```python
from build123d import *

# Parameters (mm, degrees)
CROQUIS1_R              = 2.4
CROQUIS1_R_2            = 2.1
SALIENTE_EXTRUIR1_DEPTH = 0.2
CROQUIS3_R              = 5.6
CROQUIS3_R_2            = 2.3
SALIENTE_EXTRUIR2_DEPTH = 0.1
CROQUIS5_R              = 2.4
CROQUIS5_R_2            = 2.1
SALIENTE_EXTRUIR3_DEPTH = 5


with BuildPart() as part:
    # Croquis1 → Saliente-Extruir1 (new body)
    with BuildSketch(Plane(origin=(0, 0, 0), x_dir=(1, 0, 0), z_dir=(0, 1, 0))):
        Circle(CROQUIS1_R)
        Circle(CROQUIS1_R_2, mode=Mode.SUBTRACT)
    saliente_extruir1 = extrude(amount=SALIENTE_EXTRUIR1_DEPTH)



with BuildPart() as body_2:
    # Croquis3 → Saliente-Extruir2 (new body)
    with BuildSketch(Plane.XZ):
        Circle(CROQUIS3_R)
        Circle(CROQUIS3_R_2, mode=Mode.SUBTRACT)
    saliente_extruir2 = extrude(amount=SALIENTE_EXTRUIR2_DEPTH)


with BuildPart() as part_1:
    add(part.part)

    add(body_2.part)  # Saliente-Extruir3 merges body 2
    # Croquis5 → Saliente-Extruir3 (add)
    with BuildSketch(Plane.XZ):
        Circle(CROQUIS5_R)
        Circle(CROQUIS5_R_2, mode=Mode.SUBTRACT)
    saliente_extruir3 = extrude(amount=SALIENTE_EXTRUIR3_DEPTH)

    # Simetría2: Saliente-Extruir1, Saliente-Extruir2, Saliente-Extruir3 across plane
    add(saliente_extruir1.mirror(Plane(origin=(0, -5, 0), x_dir=(0, 0, 1), z_dir=(0, -1, 0))))
    add(saliente_extruir2.mirror(Plane(origin=(0, -5, 0), x_dir=(0, 0, 1), z_dir=(0, -1, 0))))
    add(saliente_extruir3.mirror(Plane(origin=(0, -5, 0), x_dir=(0, 0, 1), z_dir=(0, -1, 0))))


solid = part_1.part
```
Input: part model. Units: mm. Frame: model coordinates. Coordinates: 2 decimals unless noted, no trailing zeros. Loops run counter-clockwise (first coordinate to the right, second up) from the corner with the lowest first, then second, coordinate; pieces in that order, holes last.
Q1. Contact query for flat-ended pins moving along their axis: pin 1 (3 mm diameter, centred on y = -8, z = -0.5, fed in from -X); pin 2 (4 mm diameter, centred on x = -3, y = -2.5, fed in from +Z); pin 3 (2 mm diameter, centred on x = -0.5, y = -6, fed in from -Z). Output: stop coordinate, or through.
Results are:
pin 1: stops at x = -2.4
pin 2: stops at z = 2.18
pin 3: stops at z = -2.4
Q2. Section A-A, the plane z = 0. Return the cut outline in (x, y), and give its area (3 significant figures).
Results are:
outline: (-5.6, -10) - (-2.4, -10) - (-2.4, -10.2) - (-2.1, -10.2) - (-2.1, 0.2) - (-2.4, 0.2) - (-2.4, 0) - (-5.6, 0) - (-5.6, -0.1) - (-2.4, -0.1) - (-2.4, -9.9) - (-5.6, -9.9) - close; (2.1, -10.2) - (2.4, -10.2) - (2.4, -10) - (5.6, -10) - (5.6, -9.9) - (2.4, -9.9) - (2.4, -0.1) - (5.6, -0.1) - (5.6, 0) - (2.4, 0) - (2.4, 0.2) - (2.1, 0.2) - close
area: 7.52 mm2
Q3. Section D-D, the plane z = 1.5. Return the cut outline in (x, y), and give its area (3 significant figures).
Results are:
outline: (-5.4, -10) - (-1.87, -10) - (-1.87, -10.2) - (-1.47, -10.2) - (-1.47, 0.2) - (-1.87, 0.2) - (-1.87, 0) - (-5.4, 0) - (-5.4, -0.1) - (-1.87, -0.1) - (-1.87, -9.9) - (-5.4, -9.9) - close; (1.47, -10.2) - (1.87, -10.2) - (1.87, -10) - (5.4, -10) - (5.4, -9.9) - (1.87, -9.9) - (1.87, -0.1) - (5.4, -0.1) - (5.4, 0) - (1.87, 0) - (1.87, 0.2) - (1.47, 0.2) - close
area: 9.81 mm2
Q4. Section B-B, the plane x = -4.5. Return the cut outline in (y, z), and give its area (3 significant figures).
Results are:
outline: (-10, -3.33) - (-9.9, -3.33) - (-9.9, 3.33) - (-10, 3.33) - close; (-0.1, -3.33) - (0, -3.33) - (0, 3.33) - (-0.1, 3.33) - close
area: 1.33 mm2
Q5. Line query: line 1 along X through (y, z) = (-7.25, 0); line 2 along Z through (x, y) = (-0.5, -6). Output: solid intervals per line, ascending.
Results are:
line 1: x = -2.4 to -2.1, 2.1 to 2.4
line 2: z = -2.35 to -2.04, 2.04 to 2.35
Q6. Section C-C, the plane y = -0.75. Return the cut outline in (x, z), and give its area (3 significant figures).
Results are:
outline: circle Ø4.8 at (0, 0); hole circle Ø4.2 at (0, 0)
area: 4.24 mm2
